CAD build for the part. Positions are in the model's coordinates, mm. A direction names the side the tool comes from. Give positions to 0.01 mm unless a question says otherwise; leave off trailing zeros. Use one line per item in the form item = value.
```python
from build123d import *

# Parameters (mm, degrees)
SKETCH_1_W               = 20
SKETCH_1_H               = 20
SKETCH_1_R               = 2
SKETCH_1_R_2             = 2.15
EXTRUDE_1_DEPTH          = 196
CUT_EXTRUDE_1_REACH      = 198.51
PATTERN_CIRCULAR_1_COUNT = 4
FILLET_1_R               = 0.3
SKETCH_4_R               = 2.5
CUT_EXTRUDE_4_DEPTH      = 198.271386673


with BuildPart() as part:
    # Sketch 1 → Extrude 1 (new body)
    with BuildSketch(Plane.XY):
        Rectangle(SKETCH_1_W, SKETCH_1_H)
        with Locations((-7, 7)):
            Circle(SKETCH_1_R, mode=Mode.SUBTRACT)
        with Locations((-7, -7)):
            Circle(SKETCH_1_R, mode=Mode.SUBTRACT)
        Circle(SKETCH_1_R_2, mode=Mode.SUBTRACT)
        with Locations((7, 7)):
            Circle(SKETCH_1_R, mode=Mode.SUBTRACT)
        with Locations((7, -7)):
            Circle(SKETCH_1_R, mode=Mode.SUBTRACT)
    extrude(amount=EXTRUDE_1_DEPTH)

    # Sketch 1_3 → Cut-Extrude 1 (cut, up to next)
    with BuildSketch(Plane.XY, mode=Mode.PRIVATE) as cut_extrude_1_sk1:
        with BuildLine():
            Line((-8.5, 2.65), (-10, 2.65))
            Line((-10, 2.65), (-10, -2.65))
            Line((-10, -2.65), (-8.5, -2.65))
            Line((-8.5, -2.65), (-8.5, -4.15))
            Line((-8.5, -4.15), (-4.503166667, -4.15))
            ThreePointArc((-4.503166667, -4.15), (-3.3, 0), (-4.503166667, 4.15))
            Line((-4.503166667, 4.15), (-8.5, 4.15))
            Line((-8.5, 4.15), (-8.5, 2.65))
        make_face()
    cut_extrude_1_tool1 = extrude(cut_extrude_1_sk1.sketch, amount=CUT_EXTRUDE_1_REACH, mode=Mode.PRIVATE) & part.part
    cut_extrude_1 = cut_extrude_1_tool1.solids().sort_by_distance((-6.606913, 0, 0))[0]
    add(cut_extrude_1, mode=Mode.SUBTRACT)

    # Pattern Circular 1: Cut-Extrude 1 ×4 about axis
    pattern_circular_1_axis = Axis((0, 0, 0), (0, 0, 1))
    for i in range(1, PATTERN_CIRCULAR_1_COUNT):
        add(cut_extrude_1.rotate(pattern_circular_1_axis, i * 360 / PATTERN_CIRCULAR_1_COUNT), mode=Mode.SUBTRACT)

    # Fillet 1
    fillet_1_edges = [part.edges().sort_by_distance(p)[0] for p in [
        (-10, -10, 98),
        (10, -10, 98),
        (10, 10, 98),
        (-10, 10, 98),
    ]]
    fillet(fillet_1_edges, radius=FILLET_1_R)

    # Sketch 4 → Cut-Extrude 4 (cut, through all)
    with BuildSketch(Plane.XZ.offset(10)):
        with Locations(Location((0, 98, 0), (0, 0, 270))):
            Circle(SKETCH_4_R)
    extrude(amount=-CUT_EXTRUDE_4_DEPTH, mode=Mode.SUBTRACT)


solid = part.part
```
1. Mould opens along X. For faces 3 (the flat face through (-10, -6, 97)), 4 (the flat face through (6, -10, 97)), 5 (the cylindrical face through (-2.44, -0.05, 98.54)) say: pulls with the +X half, pulls with the -X half, needs draft (parallel to the pull), parting line crosses it, or undercut.
Result sheet:
face_3 = pulls with the -X half
face_4 = needs draft
face_5 = undercut
2. Drop flat-ended pins along their axis: P1, Ø5, axis at x = 0, z = 84.5, coming from the -Y side; P2, Ø2, axis at y = 1.5, z = 73.5, coming from the +X side. Give the stop position or say it passes through.
Result sheet:
P1 = -3.71
P2 = 3.71
3. Tool access for faces 1 (the flat face through (-6, 10, 97)), 2 (the flat face through (-6, 4.15, 97)): list every direction of +Z, -Z, +X, -X, +Y, -Y with a clear straight run to the whole face (end or side of a thin tool).
Result sheet:
face_1 = +Z, -Z, +X, -X, +Y
face_2 = +Z, -Z
4. Cut at A-A, the plane z = 70. State how many separate pieces and enclosed holes the cut face has, then the cut area to 3 significant figures.
Result sheet:
separate_pieces = 1
enclosed_holes = 5
area = 144 mm^2
5. Drill centre lines: line 1 (Y direction, x = -7, z = 134); line 2 (Y direction, x = 0, z = 71). Where is each one in solid material? Low to high.
Result sheet:
line_1 = -10 to -9, -5 to -4.15, 4.15 to 5, 9 to 10
line_2 = -3.3 to -2.15, 2.15 to 3.3
